Part model, mm, in its own coordinate system. Coordinates: 2 decimals unless noted, no trailing zeros. Write each loop counter-clockwise with the first axis right and the second up, starting at its lowest first coordinate (ties: lowest second). Pieces come first, ordered by that corner, then holes. Notation, with made-up numbers: (16.25, -34.5) - (38.25, -34.5) arc R15 cw to (38.25, -25.5) - close; hole circle Ø10 at (-26, -24). An arc over 180 degrees is marked (long way). Write each question's results on one line, items separated by ' | '.
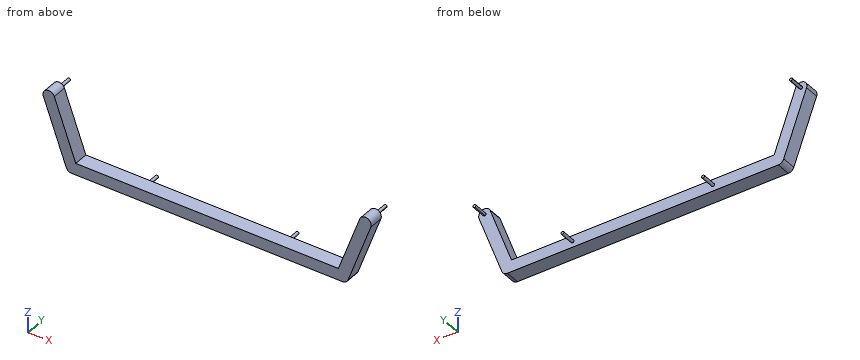
from build123d import *

# Parameters (mm, degrees)
F1_DEPTH = 50
F2_DEPTH = 25


with BuildPart() as f1:
    # F0 (on Front) → F1 (new body)
    with BuildSketch(Plane.XZ):
        with BuildLine():
            ThreePointArc((231.0551849335, -10), (223.9841171217, -7.0710678119), (221.0551849335, 0))
            ThreePointArc((221.0551849335, 0), (221.2071074034, 1.7364817767), (221.6582587257, 3.4202014333))
            Line((221.6582587257, 3.4202014333), (224.0531095514, 10))
            Line((224.0531095514, 10), (0, 10))
            ThreePointArc((0, 10), (-10, 0), (0, -10))
            Line((0, -10), (231.0551849335, -10))
        make_face()
        with BuildLine():
            ThreePointArc((122.5, 0), (120, -2.5), (117.5, 0))
            ThreePointArc((117.5, 0), (120, 2.5), (122.5, 0))
        make_face(mode=Mode.SUBTRACT)
        with BuildLine():
            Line((231.0551849335, 0), (221.0551849335, 0))
            ThreePointArc((221.0551849335, 0), (223.9841171217, -7.0710678119), (231.0551849335, -10))
            ThreePointArc((231.0551849335, -10), (236.790949297, -8.1915204429), (240.4521111414, -3.4202014333))
            ThreePointArc((240.4521111414, -3.4202014333), (240.1182628039, 4.2261826174), (234.4753863668, 9.3969262079))
            Line((234.4753863668, 9.3969262079), (231.0551849335, 0))
        make_face()
        with BuildLine():
            ThreePointArc((231.0551849335, 10), (232.7916667102, 9.8480775301), (234.4753863668, 9.3969262079))
            ThreePointArc((234.4753863668, 9.3969262079), (240.1182628039, 4.2261826174), (240.4521111414, -3.4202014333))
            Line((240.4521111414, -3.4202014333), (279.3969262079, 103.5797985667))
            ThreePointArc((279.3969262079, 103.5797985667), (273.4202014333, 116.3969262079), (260.6030737921, 110.4202014333))
            Line((260.6030737921, 110.4202014333), (224.0531095514, 10))
            Line((224.0531095514, 10), (231.0551849335, 10))
        make_face()
        with BuildLine():
            ThreePointArc((272.5, 107), (271.4339410909, 104.9521198893), (269.1449496417, 104.650768448))
            ThreePointArc((269.1449496417, 104.650768448), (268.5660589091, 109.0478801107), (272.5, 107))
        make_face(mode=Mode.SUBTRACT)
        with BuildLine():
            ThreePointArc((221.6582587257, 3.4202014333), (221.2071074034, 1.7364817767), (221.0551849335, 0))
            Line((221.0551849335, 0), (231.0551849335, 0))
            Line((231.0551849335, 0), (234.4753863668, 9.3969262079))
            ThreePointArc((234.4753863668, 9.3969262079), (232.7916667102, 9.8480775301), (231.0551849335, 10))
            Line((231.0551849335, 10), (224.0531095514, 10))
            Line((224.0531095514, 10), (221.6582587257, 3.4202014333))
        make_face()
        with BuildLine():
            ThreePointArc((272.5, 107), (268.5660589091, 109.0478801107), (269.1449496417, 104.650768448))
            ThreePointArc((269.1449496417, 104.650768448), (271.4339410909, 104.9521198893), (272.5, 107))
        make_face()
        with BuildLine():
            Line((122.5, 0), (117.5, 0))
            ThreePointArc((117.5, 0), (120, -2.5), (122.5, 0))
        make_face()
        with BuildLine():
            ThreePointArc((122.5, 0), (120, 2.5), (117.5, 0))
            Line((117.5, 0), (122.5, 0))
        make_face()
    extrude(amount=F1_DEPTH)

    # F0 (on Front) → F2 (cut)
    with BuildSketch(Plane.XZ):
        with BuildLine():
            ThreePointArc((231.0551849335, -10), (223.9841171217, -7.0710678119), (221.0551849335, 0))
            ThreePointArc((221.0551849335, 0), (221.2071074034, 1.7364817767), (221.6582587257, 3.4202014333))
            Line((221.6582587257, 3.4202014333), (224.0531095514, 10))
            Line((224.0531095514, 10), (0, 10))
            ThreePointArc((0, 10), (-10, 0), (0, -10))
            Line((0, -10), (231.0551849335, -10))
        make_face()
        with BuildLine():
            ThreePointArc((122.5, 0), (120, -2.5), (117.5, 0))
            ThreePointArc((117.5, 0), (120, 2.5), (122.5, 0))
        make_face(mode=Mode.SUBTRACT)
        with BuildLine():
            ThreePointArc((221.6582587257, 3.4202014333), (221.2071074034, 1.7364817767), (221.0551849335, 0))
            Line((221.0551849335, 0), (231.0551849335, 0))
            Line((231.0551849335, 0), (234.4753863668, 9.3969262079))
            ThreePointArc((234.4753863668, 9.3969262079), (232.7916667102, 9.8480775301), (231.0551849335, 10))
            Line((231.0551849335, 10), (224.0531095514, 10))
            Line((224.0531095514, 10), (221.6582587257, 3.4202014333))
        make_face()
        with BuildLine():
            Line((231.0551849335, 0), (221.0551849335, 0))
            ThreePointArc((221.0551849335, 0), (223.9841171217, -7.0710678119), (231.0551849335, -10))
            ThreePointArc((231.0551849335, -10), (236.790949297, -8.1915204429), (240.4521111414, -3.4202014333))
            ThreePointArc((240.4521111414, -3.4202014333), (240.1182628039, 4.2261826174), (234.4753863668, 9.3969262079))
            Line((234.4753863668, 9.3969262079), (231.0551849335, 0))
        make_face()
        with BuildLine():
            ThreePointArc((231.0551849335, 10), (232.7916667102, 9.8480775301), (234.4753863668, 9.3969262079))
            ThreePointArc((234.4753863668, 9.3969262079), (240.1182628039, 4.2261826174), (240.4521111414, -3.4202014333))
            Line((240.4521111414, -3.4202014333), (279.3969262079, 103.5797985667))
            ThreePointArc((279.3969262079, 103.5797985667), (273.4202014333, 116.3969262079), (260.6030737921, 110.4202014333))
            Line((260.6030737921, 110.4202014333), (224.0531095514, 10))
            Line((224.0531095514, 10), (231.0551849335, 10))
        make_face()
        with BuildLine():
            ThreePointArc((272.5, 107), (271.4339410909, 104.9521198893), (269.1449496417, 104.650768448))
            ThreePointArc((269.1449496417, 104.650768448), (268.5660589091, 109.0478801107), (272.5, 107))
        make_face(mode=Mode.SUBTRACT)
    extrude(amount=F2_DEPTH, mode=Mode.SUBTRACT)

    # F3: F1 across plane


with BuildPart() as f1_1:
    add(f1.part)
    add(f1.part.mirror(Plane.YZ))


with BuildPart() as f4_1:
    # F4: copy of F1
    add(f1_1.part)


solid = f1_1.part
(1) Wall check: line 1 (Z direction, x = 160, y = -43); line 2 (Y direction, x = -35, z = 8.5); line 3 (X direction, y = -33.5, z = 76). Give the ranges that are in metal, low to high. Write a range as from..to.
Return value:
line 1: z = -10..10 | line 2: y = -50..-25 | line 3: x = -269.36..-248.08, 248.08..269.36
(2) Saw through at C-C on y = -39. Write the cut outline in (x, z), then the cut area to 3 significant figures.
Return value:
outline: (-279.4, 103.58) - (-240.45, -3.42) arc R10 ccw to (-231.06, -10) - (231.06, -10) arc R10 ccw to (240.45, -3.42) - (279.4, 103.58) arc R10 ccw to (260.6, 110.42) - (224.05, 10) - (-224.05, 10) - (-260.6, 110.42) arc R10 ccw to start | area: 14,100 mm^2
(3) Saw through at D-D on x = 208. Write the cut outline in (y, z), then the cut area to 3 significant figures.
Return value:
outline: (-50, -10) - (-25, -10) - (-25, 10) - (-50, 10) - close | area: 500 mm^2
(4) Flat gauge pins, fed straight in: P1, Ø10, axis at x = 133, y = -33, coming from the +Z side; P2, Ø4, axis at y = -27.5, z = 64, coming from the +X side; P3, Ø3, axis at y = -38.5, z = 99, coming from the +X side. Where does each tip first touch, or does it go through?
Return value:
P1: stops at z = 10 | P2: stops at x = 265.72 | P3: stops at x = 278.28
(5) Saw through at A-A on y = -16. Write the cut outline in (x, z).
Return value:
outline: circle Ø5 at (-270, 107); circle Ø5 at (-120, 0); circle Ø5 at (120, 0); circle Ø5 at (270, 107)
(6) Saw through at B-B on z = 19. Write the cut outline in (x, y), then the cut area to 3 significant figures.
Return value:
outline: (-248.61, -50) - (-227.33, -50) - (-227.33, -25) - (-248.61, -25) - close; (227.33, -50) - (248.61, -50) - (248.61, -25) - (227.33, -25) - close | area: 1,060 mm^2
